from build123d import *

# Parameters (mm, degrees)
EXTRUDE_1_DEPTH     = 10
CHAMFER_2_SIZE      = 5
SKETCH_2_R          = 2.5
CUT_EXTRUDE_1_DEPTH = 30


with BuildPart() as part:
    # Эскиз1 → Бобышка-Вытянуть1 (new body)
    with BuildSketch(Plane.XY):
        with BuildLine():
            Line((0, -85), (0, 85))
            Line((0, 85), (50, 85))
            ThreePointArc((50, 85), (102.466768683, 112.312471025), (110.187404416, 170.956521648))
            ThreePointArc((110.187404416, 170.956521648), (203.389764703, 0), (110.187404416, -170.956521648))
            ThreePointArc((110.187404416, -170.956521648), (102.466768683, -112.312471025), (50, -85))
            Line((50, -85), (0, -85))
        make_face()
    extrude(amount=EXTRUDE_1_DEPTH)

    # Фаска2
    chamfer_2_edges = [part.edges().sort_by_distance(p)[0] for p in [
        (203.389764703, 0, 0),
        (203.389764703, 0, 10),
    ]]
    chamfer(chamfer_2_edges, length=CHAMFER_2_SIZE - 0.0001)  # a hair under: the kernel refuses the full size

    # Эскиз2 → Вырез-Вытянуть1 (cut)
    with BuildSketch(Plane.XY.offset(10)):
        with Locations((45, -70)):
            Circle(SKETCH_2_R)
        with Locations((70, -70)):
            Circle(SKETCH_2_R)
        with Locations((70, 70)):
            Circle(SKETCH_2_R)
        with Locations((45, 70)):
            Circle(SKETCH_2_R)
    extrude(amount=-CUT_EXTRUDE_1_DEPTH, mode=Mode.SUBTRACT)


solid = part.part
The listing builds one solid part. Answer for the finished solid, in the listing's coordinates (mm). A direction names the side the tool comes from. Give positions to 0.01 mm unless a question says otherwise; leave off trailing zeros. Loops run counter-clockwise (first coordinate to the right, second up) from the corner with the lowest first, then second, coordinate; pieces in that order, holes last. Notation, with made-up numbers: (32.5, 81) - (83.5, 81) arc R16 cw to (83.5, 103) - close; hole circle Ø6 at (68.5, 35.5). An arc over 180 degrees is marked (long way). Write each question's results on one line, items separated by ' | '.
1. For a pull along Y with two mould halves and no side action, classify faces 1 (the face through (101.97, 111.61, 4.93)), 2 (the face through (25, -85, 5)), 3 (the face through (198.61, 2.78, 9.76)), 4 (the face through (102.956, -113.021, 4.93)) as +Y half, -Y half, draft (parallel to the pull), parting line (faces both ways), or undercut.
Resolved:
face 1: undercut | face 2: -Y half | face 3: parting line | face 4: undercut
2. Consider probe 1 along Y at (x, z) = (45, 7.5); probe 2 along Y at (x, z) = (42, 5.75); probe 3 along X at (y, z) = (154.5, 3.75). Determine where each line is inside the solid, lowest interval first. Write a range as from..to.
Resolved:
probe 1: y = -85..-72.5, -67.5..67.5, 72.5..85 | probe 2: y = -85..85 | probe 3: x = 113.82..130.35
3. Find section A-A, the plane z = 2.5. Write down the section's boundary in (x, y).
Resolved:
outline: (0, -85) - (50, -85) arc R64.05 cw to (111.44, -167.15) arc R200.89 ccw to (111.44, 167.15) arc R64.05 cw to (50, 85) - (0, 85) - close; hole circle Ø5 at (45, -70); hole circle Ø5 at (45, 70); hole circle Ø5 at (70, -70); hole circle Ø5 at (70, 70)
4. Which of the six approach directions +Z, -Z, +X, -X, +Y, -Y give full straight-line access (tool end or side, diameter ignored) to faces 5 (the face through (25, 85, 5)), 6 (the face through (101, 2, 10))?
Resolved:
face 5: +Z, -Z, -X, +Y | face 6: +Z, +X, -X, +Y, -Y
5. Flat-ended cylindrical pins translate along their axes: P1, Ø4, axis at y = 0.5, z = 5.5, coming from the -X side; P2, Ø4.5, axis at x = 45, y = -70, coming from the +Z side; P3, Ø1, axis at x = 121.5, z = 9, coming from the +Y side. Find the tip coordinate at first contact, or state that the pin passes through.
Resolved:
P1: stops at x = 0 | P2: passes through | P3: stops at y = 158.83
